Read the model definition and answer for the solid it produces. Units are mm, in the model's axes. A direction names the side the tool comes from. Coordinates: 2 decimals unless noted, no trailing zeros. Order: outer loops, then holes, each group sorted by start corner. A loop starts at its lowest first (then second) coordinate and runs counter-clockwise, first axis right, second up. Notation, with made-up numbers: (-25.75, 88.25) -> (14.25, 88.25) arc R15 cw to (14.25, 112.25) -> close; hole circle Ø7 at (-9.5, -21.75). An arc over 180 degrees is marked (long way). Answer as a JSON object with one key per item and string values. Group by question number.
1) Determine the mould class of faces 1 (the cylindrical face through (-11.056, -49.787, -321.85)), 2 (the cylindrical face through (44.83, 14.12, -271.15)), 3 (the flat face through (16, -49, -100)) for opening direction X: released by +X, released by -X, zero draft, split by the parting line, or undercut.
2) A tool of negligible diameter and unlimited length cuts with its end or side. For faces 4 (the flat face through (-1, 1, 5)), 5 (the flat face through (-1, 1, 0)), from which of +Z, -Z, +X, -X, +Y, -Y can it reach the whole face along a straight path? Write none if from no direction.
3) Section C-C on z = -181.5 is taken. Determine the outline of the cut face in (x, y), and give its area (3 significant figures).
4) Consider L1, parallel to Y at x = 0, z = -355; L2, parallel to X at y = -18, z = -388. Determine where each line is inside the solid, lowest interval first.
5) Section A-A on x = 0 is taken. Determine the outline of the cut face in (y, z), and give its area (3 significant figures).
6) Given pin 1 (10 mm diameter, centred on x = -36.5, z = -478, fed in from +Y); pin 2 (3 mm diameter, centred on y = 30.5, z = -287, fed in from +X); pin 3 (12 mm diameter, centred on y = -42.5, z = -123.5, fed in from -X), each flat-ended and moving along its own axis, determine where each tip first touches the part or whether it passes through.
from build123d import *

# Parameters (mm, degrees)
F0_R     = 55
F0_R_2   = 51
F0_R_3   = 47
F1_DEPTH = 5
F2_DEPTH = 50
F3_DEPTH = 100
F4_R     = 10
F5_DEPTH = 500
F6_DEPTH = 50


with BuildPart() as f1:
    # F0 (on Top) → F1 (new body)
    with BuildSketch(Plane.XY):
        Circle(F0_R)
        Circle(F0_R_2, mode=Mode.SUBTRACT)
        Circle(F0_R_2)
        Circle(F0_R_3, mode=Mode.SUBTRACT)
        Circle(F0_R_3)
    extrude(amount=F1_DEPTH)

    # F0 (on Top) → F2 (join)
    with BuildSketch(Plane.XY):
        Circle(F0_R_2)
        Circle(F0_R_3, mode=Mode.SUBTRACT)
    extrude(amount=-F2_DEPTH)

    # F0 (on Top) → F3 (join)
    with BuildSketch(Plane.XY):
        Circle(F0_R)
        Circle(F0_R_2, mode=Mode.SUBTRACT)
    extrude(amount=-F3_DEPTH)

    # F4
    f4_edges = [f1.edges().sort_by_distance(p)[0] for p in [
        (-55, 0, 5),
    ]]
    fillet(f4_edges, radius=F4_R)

    # F5 (add): a face of the model
    f5_faces = [f1.faces().sort_by_distance(p)[0] for p in [
        (-49.5575021664, 0, -50),
    ]]
    extrude(f5_faces, amount=F5_DEPTH)

    # F6 (add): a face of the model
    f6_faces = [f1.faces().sort_by_distance(p)[0] for p in [
        (-53.4443650814, 0, -100),
    ]]
    extrude(f6_faces, amount=-F6_DEPTH)


solid = f1.part
Worked answers:
{
 "1": {"face 1": "split by the parting line", "face 2": "undercut", "face 3": "zero draft"},
 "2": {"face 4": "+Z, +X, -X, +Y, -Y", "face 5": "-Z"},
 "3": {"outline": "circle Ø102 at (0, 0); hole circle Ø94 at (0, 0)", "area": "1,230 mm²"},
 "4": {"L1": "y = -51 to -47, 47 to 51", "L2": "x = -47.72 to -43.42, 43.42 to 47.72"},
 "5": {"outline": "(-55, -100) -> (-51, -100) -> (-51, -550) -> (-47, -550) -> (-47, 0) -> (47, 0) -> (47, -550) -> (51, -550) -> (51, -100) -> (55, -100) -> (55, -5) arc R10 ccw to (45, 5) -> (-45, 5) arc R10 ccw to (-55, -5) -> close", "area": "5,710 mm²"},
 "6": {"pin 1": "stops at y = 40.11", "pin 2": "stops at x = 41.95", "pin 3": "stops at x = -35.62"}
}
